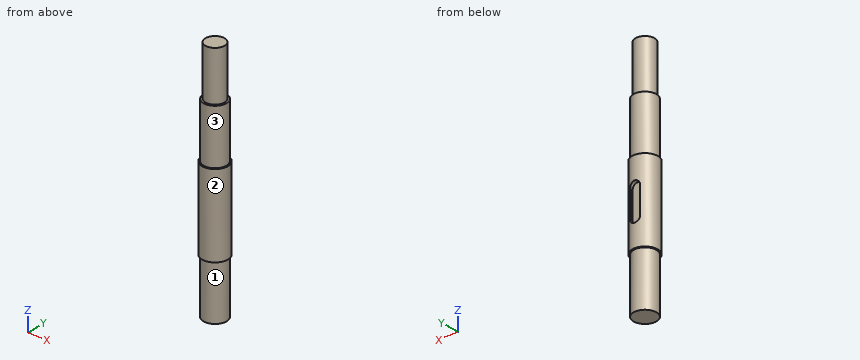
from build123d import *
from OCP.BRepAlgoAPI import BRepAlgoAPI_Cut
from OCP.TopTools import TopTools_ListOfShape

# Parameters (mm, degrees)
EXTRUDE_START       = -0.238871
SKETCH_1_R          = 3.37
EXTRUDE_1_DEPTH     = 50.000001
EXTRUDE_START_2     = 21.199419
EXTRUDE_2_DEPTH     = 7.123452
SKETCH_3_R          = 3.37
EXTRUDE_3_DEPTH     = 13
CUT_EXTRUDE_START   = -13
SKETCH_4_R          = 3.37
SKETCH_4_R_2        = 2.5
CUT_EXTRUDE_1_DEPTH = 13
CUT_EXTRUDE_START_2 = -14.3
SKETCH_5_R          = 3.37
SKETCH_5_R_2        = 3
CUT_EXTRUDE_2_DEPTH = 14.3
SKETCH_6_R          = 3.37
SKETCH_6_R_2        = 3
CUT_EXTRUDE_3_DEPTH = 14.3
CUT_EXTRUDE_4_DEPTH = 2


with BuildPart() as part:
    # 草图1 → 凸台-拉伸1 (new body)
    with BuildSketch(Plane.XY.offset(EXTRUDE_START)):
        with Locations(Location((0, 0, 0), (0, 0, 180))):
            Circle(SKETCH_1_R)
    extrude(amount=EXTRUDE_1_DEPTH)

    # 草图2 → 凸台-拉伸2 (add)
    with BuildSketch(Plane.XY.offset(EXTRUDE_START_2)):
        with BuildLine():
            Line((-1.286694662, 4.34), (1.286694662, 4.34))
            Line((1.286694662, 4.34), (1.286694662, 3.1146937))
            ThreePointArc((1.286694662, 3.1146937), (0, -3.37), (-1.286694662, 3.1146937))
            Line((-1.286694662, 3.1146937), (-1.286694662, 4.34))
        make_face()
    extrude(amount=EXTRUDE_2_DEPTH)

    # 草图3 → 凸台-拉伸3 (add)
    with BuildSketch(Plane.XY.offset(49.761129495)):
        with Locations(Location((0, 0, 0), (0, 0, 180))):
            Circle(SKETCH_3_R)
    extrude(amount=EXTRUDE_3_DEPTH)

    # 草图4 → 切除-拉伸1 (cut)
    with BuildSketch(Plane.XY.offset(62.761129495).offset(CUT_EXTRUDE_START)):
        with Locations(Location((0, 0, 0), (0, 0, 180))):
            Circle(SKETCH_4_R)
        Circle(SKETCH_4_R_2, mode=Mode.SUBTRACT)
    extrude(amount=CUT_EXTRUDE_1_DEPTH, mode=Mode.SUBTRACT)

    # 草图5 → 切除-拉伸2 (cut)
    with BuildSketch(Plane.XY.offset(49.761129495).offset(CUT_EXTRUDE_START_2)):
        with Locations(Location((0, 0, 0), (0, 0, 180))):
            Circle(SKETCH_5_R)
        Circle(SKETCH_5_R_2, mode=Mode.SUBTRACT)
    extrude(amount=CUT_EXTRUDE_2_DEPTH, mode=Mode.SUBTRACT)


with BuildPart() as cut_extrude_3_tool:
    # 草图6 → 切除-拉伸3 (new body)
    with BuildSketch(Plane(origin=(0, 0, -0.238870505), x_dir=(-1, 0, 0), z_dir=(0, 0, -1))):
        Circle(SKETCH_6_R)
        with Locations(Location((0, 0, 0), (0, 0, 180))):
            Circle(SKETCH_6_R_2, mode=Mode.SUBTRACT)
    extrude(amount=-CUT_EXTRUDE_3_DEPTH)


with BuildPart() as part_1:
    add(part.part)

    # 切除-拉伸3: cut by cut_extrude_3_tool, with a tolerance
    cut_extrude_3_stock = TopTools_ListOfShape()
    cut_extrude_3_stock.Append(part_1.part.wrapped)
    cut_extrude_3_tools = TopTools_ListOfShape()
    cut_extrude_3_tools.Append(cut_extrude_3_tool.part.wrapped)
    cut_extrude_3_cut = BRepAlgoAPI_Cut()
    cut_extrude_3_cut.SetArguments(cut_extrude_3_stock)
    cut_extrude_3_cut.SetTools(cut_extrude_3_tools)
    cut_extrude_3_cut.SetFuzzyValue(0.00001)
    cut_extrude_3_cut.Build()
    add(Compound.cast(cut_extrude_3_cut.Shape()).solids(), mode=Mode.REPLACE)

    # 草图7 → 切除-拉伸4 (cut)
    with BuildSketch(Plane(origin=(0, 4.34, 0), x_dir=(1, 0, 0), z_dir=(0, 1, 0))):
        with BuildLine():
            Line((-1.286694662, -28.322870736), (-1.286694662, -21.199418736))
            ThreePointArc((-1.286694662, -21.199418736), (0, -19.912724074), (1.286694662, -21.199418736))
            Line((1.286694662, -21.199418736), (1.286694662, -28.322870736))
            ThreePointArc((1.286694662, -28.322870736), (0, -29.609565398), (-1.286694662, -28.322870736))
        make_face()
    extrude(amount=-CUT_EXTRUDE_4_DEPTH, mode=Mode.SUBTRACT)


solid = part_1.part
The listing builds one solid part. Answer for the finished solid, in the listing's coordinates (mm). Face numbers are marked on the shaded views. A direction names the side the tool comes from. Coordinates: 2 decimals unless noted, no trailing zeros. Loops run counter-clockwise (first coordinate to the right, second up) from the corner with the lowest first, then second, coordinate; pieces in that order, holes last. Notation, with made-up numbers: M 86.25,55.5 L 115.25,55.5 A16 cw 115.25,60.5 Z; hole C 36.5,25.5 d4. An arc over 180 degrees is marked long. Answer in a Markdown table with one row per item.
1) Find the intervals of material crossed by probe 1 along Z at (x, y) = (-2, -1.75); probe 2 along Y at (x, z) = (0.25, 13.5); probe 3 along Z at (x, y) = (-2.5, 1.75), in increasing order.
Answers below:
| item | result |
|---|---|
| probe 1 | -0.24 to 49.76 |
| probe 2 | -2.99 to 2.99 |
| probe 3 | 14.06 to 35.46 |
2) Which of the six approach directions +Z, -Z, +X, -X, +Y, -Y give full straight-line access (tool end or side, diameter ignored) to the marked faces 1, 2 and 3?
Answers below:
| item | result |
|---|---|
| face 1 | -Z |
| face 2 | +Z, -Z |
| face 3 | +Z |
3) Find section C-C (z = 55.5). Determine the outline of the cut face in (x, y).
Answers below:
| item | result |
|---|---|
| outline | C 0,0 d5 |
4) Given pin 1 (1 mm diameter, centred on y = -2.5, z = 34, fed in from +X); pin 2 (0.8 mm diameter, centred on x = 0, z = 24, fed in from +Y); pin 3 (1 mm diameter, centred on y = 1.5, z = 26.5, fed in from -X); pin 4 (3 mm diameter, centred on y = 0.5, z = 21, fed in from +X), each flat-ended and moving along its own axis, determine where each tip first touches the part or whether it passes through.
Answers below:
| item | result |
|---|---|
| pin 1 | x = 2.71 |
| pin 2 | y = 2.34 |
| pin 3 | x = -3.22 |
| pin 4 | x = 3.37 |
5) Find section A-A (x = 0). Determine the outline of the cut face in (y, z).
Answers below:
| item | result |
|---|---|
| outline | M -3.37,14.06 L -3,14.06 L -3,-0.24 L 3,-0.24 L 3,14.06 L 3.37,14.06 L 3.37,19.91 L 2.34,19.91 L 2.34,29.61 L 3.37,29.61 L 3.37,35.46 L 3,35.46 L 3,49.76 L 2.5,49.76 L 2.5,62.76 L -2.5,62.76 L -2.5,49.76 L -3,49.76 L -3,35.46 L -3.37,35.46 Z |
6) Find section D-D (z = 45.5). Determine the outline of the cut face in (x, y), then the cut area to 3 significant figures.
Answers below:
| item | result |
|---|---|
| outline | C 0,0 d6 |
| area | 28.3 mm^2 |
7) Find section B-B (y = 0). Determine the outline of the cut face in (x, z), then the cut area to 3 significant figures.
Answers below:
| item | result |
|---|---|
| outline | M -3.37,14.06 L -3,14.06 L -3,-0.24 L 3,-0.24 L 3,14.06 L 3.37,14.06 L 3.37,35.46 L 3,35.46 L 3,49.76 L 2.5,49.76 L 2.5,62.76 L -2.5,62.76 L -2.5,49.76 L -3,49.76 L -3,35.46 L -3.37,35.46 Z |
| area | 381 mm^2 |
